Geometry: final body of the model. Coordinates: model frame, mm. A direction names the side the tool comes from. Coordinates: 2 decimals unless noted, no trailing zeros. Loops run counter-clockwise (first coordinate to the right, second up) from the corner with the lowest first, then second, coordinate; pieces in that order, holes last. Notation, with made-up numbers: (-3, 77) - (18, 77) arc R21 ccw to (18, 94) - close; hole circle Ø4 at (-27, -36.5). An arc over 180 degrees is marked (long way). Return JSON: item names as keys, results as strings.
from build123d import *

# Parameters (mm, degrees)
CUT_EXTRUDE1_REACH = 40.962
SKETCH2_W          = 9.385810436
SKETCH2_H          = 34.336908986
SKETCH2_W_2        = 16.426678561
SKETCH2_H_2        = 32.704594128
CUT_EXTRUDE2_REACH = 33.801
SKETCH3_R          = 1.7859375


with BuildPart() as part:
    # Sketch1 → Revolve2 (revolve)
    with BuildSketch(Plane.XY, mode=Mode.PRIVATE) as revolve2_sk:
        Polygon((0, 0), (9.525, 0), (9.525, 3.175), (3.175, 3.175), (3.175, 10.16), (-1.27, 10.16), (-1.27, 6.985), (0, 6.985), align=None)
    revolve(revolve2_sk.sketch.rotate(Axis((-10.9982, 23.074413867, 0), (0, -1, 0)), 180), axis=Axis((-10.9982, 23.074413867, 0), (0, -1, 0)))

    # Cut-Extrude1: up to this face of the body (flat: up to its plane)
    cut_extrude1_end = Plane(part.part.faces().sort_by_distance((0.580483756, 0, 0))[0])
    # Sketch2 → Cut-Extrude1 (cut, up to the picked face)
    with BuildSketch(Plane(origin=(0, 10.16, 0), x_dir=(1, 0, 0), z_dir=(0, 1, 0)), mode=Mode.PRIVATE) as cut_extrude1_sk1:
        with Locations((-27.959305218, 0)):
            Rectangle(SKETCH2_W, SKETCH2_H)
    cut_extrude1_tool1 = split(extrude(cut_extrude1_sk1.sketch, amount=-CUT_EXTRUDE1_REACH, mode=Mode.PRIVATE), bisect_by=cut_extrude1_end, keep=Keep.BOTH, mode=Mode.PRIVATE)
    # Sketch2 → Cut-Extrude1 (cut, up to the picked face)
    with BuildSketch(Plane(origin=(0, 10.16, 0), x_dir=(1, 0, 0), z_dir=(0, 1, 0)), mode=Mode.PRIVATE) as cut_extrude1_sk2:
        with Locations((9.483339281, 0)):
            Rectangle(SKETCH2_W_2, SKETCH2_H_2)
    cut_extrude1_tool2 = split(extrude(cut_extrude1_sk2.sketch, amount=-CUT_EXTRUDE1_REACH, mode=Mode.PRIVATE), bisect_by=cut_extrude1_end, keep=Keep.BOTH, mode=Mode.PRIVATE)
    add(cut_extrude1_tool1.solids().sort_by(Axis((-27.959305, 10.16, 0), (0, -1, 0)))[0], mode=Mode.SUBTRACT)
    add(cut_extrude1_tool2.solids().sort_by(Axis((9.483339, 10.16, 0), (0, -1, 0)))[0], mode=Mode.SUBTRACT)

    # Sketch3 → Cut-Extrude2 (cut, up to next)
    with BuildSketch(Plane(origin=(0, 3.175, 0), x_dir=(1, 0, 0), z_dir=(0, 1, 0)), mode=Mode.PRIVATE) as cut_extrude2_sk1:
        with Locations(Location((-10.9982, 17.145, 0), (0, 0, 180))):
            Circle(SKETCH3_R)
    cut_extrude2_tool1 = extrude(cut_extrude2_sk1.sketch, amount=-CUT_EXTRUDE2_REACH, mode=Mode.PRIVATE) & part.part
    # Sketch3 → Cut-Extrude2 (cut, up to next)
    with BuildSketch(Plane(origin=(0, 3.175, 0), x_dir=(1, 0, 0), z_dir=(0, 1, 0)), mode=Mode.PRIVATE) as cut_extrude2_sk2:
        with Locations(Location((-10.9982, -17.145, 0), (0, 0, 180))):
            Circle(SKETCH3_R)
    cut_extrude2_tool2 = extrude(cut_extrude2_sk2.sketch, amount=-CUT_EXTRUDE2_REACH, mode=Mode.PRIVATE) & part.part
    add(cut_extrude2_tool1.solids().sort_by_distance((-10.9982, 3.175, -17.145))[0], mode=Mode.SUBTRACT)
    add(cut_extrude2_tool2.solids().sort_by_distance((-10.9982, 3.175, 17.145))[0], mode=Mode.SUBTRACT)


solid = part.part
Item 1: Ray query, probe 1 along Z at (x, y) = (-11.25, 1.75); probe 2 along Y at (x, z) = (-12, 19.5) (3 decimals); probe 3 along X at (y, z) = (5.5, 6). Return the intervals inside material, ascending. Write a range as from..to.
Worked out:
{"probe 1": "-20.52..-18.91, -15.38..-11, 11..15.38, 18.91..20.52", "probe 2": "0..3.175", "probe 3": "-23.27..-20.22, -1.78..1.27"}
Item 2: Reachability of faces 1 (the face through (-16.07, 3.44, 9.76)), 2 (the face through (-23.266, 4, 0)), 3 (the face through (-11, 3.175, 15)), 4 (the face through (-8, 3.175, -15)) from +Z, -Z, +X, -X, +Y, -Y: full face, straight path, thin tool, end or side. Return the list, or none.
Worked out:
{"face 1": "-Y", "face 2": "+Z, -Z, -X, +Y, -Y", "face 3": "+Z, +Y", "face 4": "-Z, +Y"}
Item 3: Section query D-D, the plane z = 4.5. Return loops of the section in (x, y) (3 decimals).
Worked out:
{"outline": "(-23.266, 0) - (-21.034, 0) - (-21.034, 6.985) - (-19.623, 6.985) - (-19.623, 10.16) - (-23.266, 10.16) - close; (-2.373, 6.985) - (-0.963, 6.985) - (-0.963, 0) - (1.27, 0) - (1.27, 10.16) - (-2.373, 10.16) - close"}
Item 4: Section query C-C, the plane y = 7.75. Return loops of the section in (x, z), and give its area (3 significant figures).
Worked out:
{"outline": "(-23.27, -7.1) arc R14.17 ccw to (1.27, -7.1) - (1.27, 7.1) arc R14.17 ccw to (-23.27, 7.1) - close; hole circle Ø19.46 at (-11, 0)", "area": "297 mm^2"}
Item 5: First-contact query: pin 1 Ø5 at (y, z) = (6.5, 5.5) entering from +X; pin 2 Ø8 at (x, z) = (-7.5, -0.5) entering from -Y. Flat tips, straight axial feed; report the tip coordinate or a pass-through.
Worked out:
{"pin 1": "x = 1.27", "pin 2": "through"}
Item 6: Section query A-A, the plane z = 0. Return loops of the section in (x, y) (3 decimals).
Worked out:
{"outline": "(-23.266, 0) - (-21.996, 0) - (-21.996, 6.985) - (-20.726, 6.985) - (-20.726, 10.16) - (-23.266, 10.16) - close; (-1.27, 6.985) - (0, 6.985) - (0, 0) - (1.27, 0) - (1.27, 10.16) - (-1.27, 10.16) - close"}
Item 7: Mould query, pull axis Z, two halves, no side actions, for faces 5 (the face through (-11.21, 6.72, -14.17)), 6 (the face through (-9.68, 1.61, -15.94)), 7 (the face through (-22, 0, -5)), 8 (the face through (1.27, 4, 0)). Classes: +Z half, -Z half, draft (parallel to the pull), parting line (faces both ways), or undercut.
Worked out:
{"face 5": "-Z half", "face 6": "undercut", "face 7": "draft", "face 8": "undercut"}
Item 8: Section query B-B, the plane x = -4.75. Return loops of the section in (y, z) (3 decimals).
Worked out:
{"outline": "(0, -19.549) - (3.175, -19.549) - (3.175, -12.722) - (10.16, -12.722) - (10.16, -7.456) - (6.985, -7.456) - (6.985, -9.051) - (0, -9.051) - close; (0, 9.051) - (6.985, 9.051) - (6.985, 7.456) - (10.16, 7.456) - (10.16, 12.722) - (3.175, 12.722) - (3.175, 19.549) - (0, 19.549) - close"}
